```python
from build123d import *

# Parameters (mm, degrees)
BOSS_EXTRUDE1_DEPTH = 10
CUT_EXTRUDE2_DEPTH  = 6.5
FILLET1_R           = 0.5
FILLET2_R           = 0.5


with BuildPart() as part:
    # Sketch1 → Boss-Extrude1 (new body)
    with BuildSketch(Plane.XY):
        Polygon((-2.5, -4.047619048), (2.5, -4.047619048), (4.5, -1.047619048), (4.5, -0.047619048), (2.5, -0.047619048), (2.5, 1.452380952), (-2.5, 1.452380952), (-2.5, -0.047619048), (-4.5, -0.047619048), (-4.5, -1.047619048), align=None)
    extrude(amount=BOSS_EXTRUDE1_DEPTH)

    # Sketch4 → Cut-Extrude2 (cut, through all)
    with BuildSketch(Plane(origin=(0, 1.452380952, 0), x_dir=(1, 0, 0), z_dir=(0, 1, 0))):
        Polygon((-1.021105314, -4.986458601), (-0.021105314, -3.986458601), (0.978894686, -4.986458601), (-0.021105314, -5.986458601), align=None)
    extrude(amount=-CUT_EXTRUDE2_DEPTH, mode=Mode.SUBTRACT)

    # Fillet1
    fillet1_edges = [part.edges().sort_by_distance(p)[0] for p in [
        (2.5, -4.047619048, 5),
        (-2.5, -4.047619048, 5),
        (-4.5, -1.047619048, 5),
        (-4.5, -0.047619048, 5),
        (-2.5, 1.452380952, 5),
        (2.5, 1.452380952, 5),
        (4.5, -0.047619048, 5),
        (4.5, -1.047619048, 5),
    ]]
    fillet(fillet1_edges, radius=FILLET1_R)

    # Fillet2
    fillet2_edges = [part.edges().sort_by_distance(p)[0] for p in [
        (2.5, 0.452380952, 10),
        (-3.25, -0.047619048, 10),
        (3.532229208, -2.499275236, 10),
        (0, -4.047619048, 10),
        (4.5, -0.721925138, 10),
        (3.25, -0.047619048, 10),
        (0, 1.452380952, 10),
        (-2.5, 0.452380952, 10),
        (-4.5, -0.721925138, 10),
        (-3.532229208, -2.499275236, 10),
        (-2.353553391, 1.305934343, 10),
        (-4.353553391, -0.194065657, 10),
        (-4.478546013, -1.041123303, 10),
        (2.353553391, 1.305934343, 10),
        (4.353553391, -0.194065657, 10),
        (4.478546013, -1.041123303, 10),
        (-2.468337084, -3.988456347, 10),
        (2.468337084, -3.988456347, 10),
    ]]
    fillet(fillet2_edges, radius=FILLET2_R)


solid = part.part
```
Verification items for the finished model (mm, model axes). A direction names the side the tool comes from. Round coordinates to 2 decimals unless told otherwise and drop trailing zeros. Write each loop counter-clockwise with the first axis right and the second up, starting at its lowest first coordinate (ties: lowest second). Pieces come first, ordered by that corner, then holes. Notation, with made-up numbers: (14.5, 42.5) -> (22.5, 42.5) arc R23 ccw to (22.5, 67.5) -> close; hole circle Ø4 at (16, 22.5). An arc over 180 degrees is marked (long way). Write each question's results on one line, items separated by ' | '. Start each with the question number.
1. Depth check by flat-ended pin: P1, Ø0.5, axis at y = 0.5, z = 4.5, coming from the +X side. Enter the tip coordinate at first touch or a pass-through.
2. Material ranges on probe 1 along X at (y, z) = (1.1, 5.5); probe 2 along X at (y, z) = (0.2, 8.75); probe 3 along X at (y, z) = (-0.95, 3.75), recorded low to high. Write a range as from..to.
3. Cross-section at C-C (z = 3.5). Enter the section's corners in (x, y), then the cut area to 3 significant figures.
4. Cross-section at B-B (y = -0.25). Enter the section's corners in (x, z).
5. Draft check along Z on faces 1 (the flat face through (0, -1, 10)), 2 (the flat face through (0, -1, 0)), 3 (the flat face through (-3.545, -2.481, 4.684)), 4 (the flat face through (-0.528, -1.259, 4.493)). Enter one of: +Z half, -Z half, draft (parallel to the pull), parting line (faces both ways), or undercut.
6. Set-up check for faces 5 (the flat face through (-0.514, -1.259, 5.493)), 6 (the flat face through (3, -0.048, 5)), 7 (the flat face through (-2.5, 0.5, 4.7)), 8 (the flat face through (3.52, -2.52, 4.68)): record each of +Z, -Z, +X, -X, +Y, -Y from which the full face is reachable in a straight line by a thin tool's end or side.
7. Cross-section at A-A (z = 5.25). Enter the section's corners in (x, y), then the cut area to 3 significant figures.
Solutions:
1) P1: stops at x = 2.5
2) probe 1: x = -2.48..-0.51, 0.47..2.48 | probe 2: x = -2.5..2.5 | probe 3: x = -4.5..4.5
3) outline: (-4.5, -0.9) arc R0.5 ccw to (-4.42, -1.17) -> (-2.65, -3.82) arc R0.5 ccw to (-2.23, -4.05) -> (2.23, -4.05) arc R0.5 ccw to (2.65, -3.82) -> (4.42, -1.17) arc R0.5 ccw to (4.5, -0.9) -> (4.5, -0.55) arc R0.5 ccw to (4, -0.05) -> (2.5, -0.05) -> (2.5, 0.95) arc R0.5 ccw to (2, 1.45) -> (-2, 1.45) arc R0.5 ccw to (-2.5, 0.95) -> (-2.5, -0.05) -> (-4, -0.05) arc R0.5 ccw to (-4.5, -0.55) -> close | area: 37.3 mm2
4) outline: (-4.4, 0) -> (4.4, 0) -> (4.4, 9.5) arc R0.4 ccw to (4, 9.9) -> (2.3, 9.9) arc R0.5 ccw to (2, 10) -> (-2, 10) arc R0.5 ccw to (-2.3, 9.9) -> (-4, 9.9) arc R0.4 ccw to (-4.4, 9.5) -> close; hole (-1.02, 4.99) -> (-0.02, 3.99) -> (0.98, 4.99) -> (-0.02, 5.99) -> close
5) face 1: +Z half | face 2: -Z half | face 3: draft | face 4: undercut
6) face 5: +Y, -Y | face 6: +Z, -Z, +X, +Y | face 7: +Z, -Z, -X, +Y | face 8: +Z, -Z, +X, -Y
7) outline: (-4.5, -0.9) arc R0.5 ccw to (-4.42, -1.17) -> (-2.65, -3.82) arc R0.5 ccw to (-2.23, -4.05) -> (-0.76, -4.05) -> (-0.76, 1.45) -> (-2, 1.45) arc R0.5 ccw to (-2.5, 0.95) -> (-2.5, -0.05) -> (-4, -0.05) arc R0.5 ccw to (-4.5, -0.55) -> close; (0.72, -4.05) -> (2.23, -4.05) arc R0.5 ccw to (2.65, -3.82) -> (4.42, -1.17) arc R0.5 ccw to (4.5, -0.9) -> (4.5, -0.55) arc R0.5 ccw to (4, -0.05) -> (2.5, -0.05) -> (2.5, 0.95) arc R0.5 ccw to (2, 1.45) -> (0.72, 1.45) -> close | area: 29.2 mm2
